For this review, take the finished solid that the model builds, in its own axes (mm). A direction names the side the tool comes from. Coordinates: 2 decimals unless noted, no trailing zeros. Loops run counter-clockwise (first coordinate to the right, second up) from the corner with the lowest first, then second, coordinate; pieces in that order, holes last. Notation, with made-up numbers: (21, -4.5) - (57, -4.5) arc R35 cw to (57, 29.5) - close; hole circle Ø1 at (41.5, 47). An arc over 180 degrees is marked (long way). Answer as a JSON object with one key per item and string values. Group by question number.
Item 1: Mouldability with a two-part tool opening along Y and no side actions: class faces 1 (the flat face through (0, 23, 24)), 2 (the cylindrical face through (-15.97, -22.4, 15.21)), 3 (the flat face through (17, 0, 27.6)) as released by +Y, released by -Y, zero draft, split by the parting line, or undercut.
Item 2: We need section C-C (x = 0). State how many separate pieces and enclosed holes the cut face has, then the cut area to 3 significant figures.
Item 3: We need section D-D (y = -2). Give the boundary of the cut face in (x, z), then the cut area to 3 significant figures.
Item 4: Clearance check with flat-ended pins moving along their axes: pin 1 (0.6 mm diameter, centred on x = -16.5, y = 0, fed in from -Z); pin 2 (1 mm diameter, centred on y = -14.5, z = 11, fed in from +X); pin 3 (0.6 mm diameter, centred on x = 16.5, y = 0.5, fed in from +Z); pin 4 (2.5 mm diameter, centred on y = 23, z = 10.5, fed in from +X). State where each tip first meets the part, or that it passes through.
Item 5: We need section B-B (y = 15). Give the boundary of the cut face in (x, z).
Item 6: We need section A-A (x = 8.5). Give the boundary of the cut face in (y, z), then the cut area to 3 significant figures.
Item 7: To check wall thickness, follow line 1 (Z direction, x = 0, y = -23); line 2 (Y direction, x = 12, z = 28.25); line 3 (X direction, y = -14.5, z = 22.25). State the ranges of each line that lie inside material, in increasing order.
Item 8: Tool access review of faces 4 (the flat face through (-16, 5, 15)), 5 (the flat face through (0, 22.7, 26)), 6 (the flat face through (17, 0, 2.4)), 7 (the flat face through (0, 23, 27.6)), 8 (the flat face through (17, 0, 20)): name each direction out of +Z, -Z, +X, -X, +Y, -Y from which nothing blocks a thin tool from reaching the whole face with its end or side.
from build123d import *

# Parameters (mm, degrees)
F0_W      = 1.2
F0_H      = 10
F0_W_2    = 10
F0_H_2    = 1.2
F1_DEPTH  = 30
F2_W      = 10
F2_H      = 4
F3_DEPTH  = 47.801
F4_W      = 10
F4_H      = 4
F5_DEPTH  = 34.801
F6_W      = 10
F6_H      = 1.2
F6_W_2    = 1.2
F6_H_2    = 10
F7_DEPTH  = 2.4
F8_DEPTH  = 2.4
F9_R      = 5
F2_R      = 1.5
F10_DEPTH = 1.2
F11_R     = 2.5
F12_DEPTH = 1.2
F4_R      = 1.5
F13_DEPTH = 34.801


with BuildPart() as f1:
    # F0 (on Top) → F1 (new body)
    with BuildSketch(Plane.XY):
        Polygon((15, -5), (15, -21.5), (5, -21.5), (5, -22.7), (5, -23.9), (17.4, -23.9), (17.4, -5), (16.2, -5), align=None)
        with Locations((16.8, 0)):
            Rectangle(F0_W, F0_H)
        Polygon((15, 5), (16.2, 5), (17.4, 5), (17.4, 23.9), (5, 23.9), (5, 22.7), (5, 21.5), (15, 21.5), align=None)
        with Locations((0, 23.3)):
            Rectangle(F0_W_2, F0_H_2)
        Polygon((-17.4, 23.9), (-17.4, 5), (-16.2, 5), (-15, 5), (-15, 21.5), (-5, 21.5), (-5, 22.7), (-5, 23.9), align=None)
        Polygon((-5, -23.9), (-5, -22.7), (-5, -21.5), (-15, -21.5), (-15, -5), (-16.2, -5), (-17.4, -5), (-17.4, -23.9), align=None)
        with Locations((0, -23.3)):
            Rectangle(F0_W_2, F0_H_2)
        with Locations((-16.8, 0)):
            Rectangle(F0_W, F0_H)
    extrude(amount=F1_DEPTH)

    # F2 (on face) → F3 (cut, through all)
    with BuildSketch(Plane.XZ.offset(23.9)):
        with Locations((0, 22)):
            Rectangle(F2_W, F2_H)
        with Locations((0, 8)):
            Rectangle(F2_W, F2_H)
    extrude(amount=-F3_DEPTH, mode=Mode.SUBTRACT)

    # F4 (on face) → F5 (cut, through all)
    with BuildSketch(Plane(origin=(-17.4, 0, 0), x_dir=(0, -1, 0), z_dir=(-1, 0, 0))):
        with Locations((0, 22)):
            Rectangle(F4_W, F4_H)
        with Locations((0, 8)):
            Rectangle(F4_W, F4_H)
    extrude(amount=-F5_DEPTH, mode=Mode.SUBTRACT)

    # F6 (on face) → F7 (cut)
    with BuildSketch(Plane.XY.offset(30)):
        with Locations((0, 23.3)):
            Rectangle(F6_W, F6_H)
        with Locations((16.8, 0)):
            Rectangle(F6_W_2, F6_H_2)
        with Locations((-16.8, 0)):
            Rectangle(F6_W_2, F6_H_2)
        with Locations((0, -23.3)):
            Rectangle(F6_W, F6_H)
    extrude(amount=-F7_DEPTH, mode=Mode.SUBTRACT)

    # F0 (on Top) → F8 (cut)
    with BuildSketch(Plane.XY):
        with Locations((16.8, 0)):
            Rectangle(F0_W, F0_H)
        with Locations((0, 23.3)):
            Rectangle(F0_W_2, F0_H_2)
        with Locations((0, -23.3)):
            Rectangle(F0_W_2, F0_H_2)
        with Locations((-16.8, 0)):
            Rectangle(F0_W, F0_H)
    extrude(amount=F8_DEPTH, mode=Mode.SUBTRACT)

    # F9
    f9_edges = [f1.edges().sort_by_distance(p)[0] for p in [
        (-17.4, -23.9, 15),
        (-17.4, 23.9, 15),
        (17.4, -23.9, 15),
        (17.4, 23.9, 15),
    ]]
    fillet(f9_edges, radius=F9_R)

    # F2 (on face) → F10 (cut, through all)
    with BuildSketch(Plane.XZ.offset(23.9)):
        with Locations((0, 15)):
            Circle(F2_R)
    extrude(amount=-F10_DEPTH, mode=Mode.SUBTRACT)

    # F11 (on face) → F12 (cut, through all)
    with BuildSketch(Plane(origin=(0, 23.9, 0), x_dir=(-1, 0, 0), z_dir=(0, 1, 0))):
        with Locations((0, 15)):
            Circle(F11_R)
    extrude(amount=-F12_DEPTH, mode=Mode.SUBTRACT)

    # F4 (on face) → F13 (cut, through all)
    with BuildSketch(Plane(origin=(-17.4, 0, 0), x_dir=(0, -1, 0), z_dir=(-1, 0, 0))):
        with Locations((-15, 10)):
            Circle(F4_R)
        with Locations((15, 10)):
            Circle(F4_R)
    extrude(amount=-F13_DEPTH, mode=Mode.SUBTRACT)


solid = f1.part
Check sheet entries:
{
 "1": {"face 1": "zero draft", "face 2": "released by -Y", "face 3": "undercut"},
 "2": {"separate pieces": "8", "enclosed holes": "0", "area": "31.7 mm2"},
 "3": {"outline": "(-17.4, 2.4) - (-16.2, 2.4) - (-16.2, 6) - (-17.4, 6) - close; (-17.4, 10) - (-16.2, 10) - (-16.2, 20) - (-17.4, 20) - close; (-17.4, 24) - (-16.2, 24) - (-16.2, 27.6) - (-17.4, 27.6) - close; (16.2, 2.4) - (17.4, 2.4) - (17.4, 6) - (16.2, 6) - close; (16.2, 10) - (17.4, 10) - (17.4, 20) - (16.2, 20) - close; (16.2, 24) - (17.4, 24) - (17.4, 27.6) - (16.2, 27.6) - close", "area": "41.3 mm2"},
 "4": {"pin 1": "stops at z = 2.4", "pin 2": "stops at x = 17.4", "pin 3": "stops at z = 27.6", "pin 4": "stops at x = 16.51"},
 "5": {"outline": "(-17.4, 0) - (-15, 0) - (-15, 8.5) - (-17.4, 8.5) - close; (-17.4, 11.5) - (-15, 11.5) - (-15, 30) - (-17.4, 30) - close; (15, 0) - (17.4, 0) - (17.4, 8.5) - (15, 8.5) - close; (15, 11.5) - (17.4, 11.5) - (17.4, 30) - (15, 30) - close"},
 "6": {"outline": "(-23.9, 0) - (-21.5, 0) - (-21.5, 30) - (-23.9, 30) - close; (21.5, 0) - (23.9, 0) - (23.9, 30) - (21.5, 30) - close", "area": "144 mm2"},
 "7": {"line 1": "z = 2.4 to 6, 10 to 13.5, 16.5 to 20, 24 to 27.6", "line 2": "y = -23.9 to -21.5, 21.5 to 23.9", "line 3": "x = -17.4 to -15, 15 to 17.4"},
 "8": {"face 4": "none", "face 5": "+Z, -Z", "face 6": "-Z, +X, -X", "face 7": "+Z, +Y, -Y", "face 8": "+X, -X"}
}
